Here's how the part is built. I have some questions about the finished solid (model axes, mm). A direction names the side the tool comes from. Coordinates: 2 decimals unless noted, no trailing zeros. Order: outer loops, then holes, each group sorted by start corner. A loop starts at its lowest first (then second) coordinate and runs counter-clockwise, first axis right, second up. Notation, with made-up numbers: (-12, 89) - (43, 89) arc R16 ccw to (43, 115) - close; hole circle Ø11 at (-31, 43.5). An arc over 180 degrees is marked (long way). Answer in a Markdown table with one row per item. Add a question column.
Item 1: I want a section at A-A (z = 113). Please give me the cut outline in (x, y).
Item 2: If I drill on line 1 along Z through (x, y) = (14.5, -1.5); line 2 along X through (y, z) = (-8.75, 84.4); line 3 along Y through (x, z) = (17.5, 31), over which ranges is the centre line in solid material (lowest first)? Write a range as from..to.
Item 3: Will these pins go through, and if not, where does the flat tip stop? pin 1 Ø3 at (x, y) = (15.75, -16.25) entering from +Z; pin 2 Ø5 at (x, y) = (19, 11) entering from +Z; pin 3 Ø6.5 at (x, z) = (13, 97.5) entering from +Y.
Item 4: On a 3-axis mill with a long thin cutter (end or side, diameter ignored), from which of +Z, -Z, +X, -X, +Y, -Y can I reach the whole of each face in a straight line? I mean faces 4 (the cylindrical face through (15.33, 6.297, -72.859)), 5 (the cylindrical face through (20.01, 17.95, 70.2)), 6 (the flat face through (14, 11.5, -65)), 7 (the flat face through (23.028, 20.996, -104.866)). Say none if no direction works.
Item 5: Thinking about a two-plate mould opening in Z: for faces 1 (the flat face through (15.5, 12, 102)), 2 (the cylindrical face through (22.972, 23.75, 76.245)), 3 (the flat face through (16, 2, 130)), which applies, +Z half, -Z half, draft (parallel to the pull), parting line (faces both ways), or undercut?
```python
from build123d import *

# Parameters (mm, degrees)
BOSS_EXTRUDE1_DEPTH      = 25
CUT_EXTRUDE1_DEPTH       = 4
FILLET1_R                = 4
FILLET2_R                = 10
FILLET3_R                = 5
FILLET4_R                = 3
BOSS_EXTRUDE2_DEPTH      = 3
BOSS_EXTRUDE2_DEPTH_BACK = 3
FILLET5_R                = 3
SKETCH6_W                = 13
SKETCH6_H                = 14
BOSS_EXTRUDE3_DEPTH      = 20
BOSS_EXTRUDE4_DEPTH      = 20
SKETCH9_W                = 13
SKETCH9_H                = 2
BOSS_EXTRUDE5_DEPTH      = 8
SKETCH7_W                = 13
SKETCH7_H                = 2
CUT_EXTRUDE2_DEPTH       = 5
SKETCH11_R               = 1.6
CUT_EXTRUDE3_DEPTH       = 19
CUT_EXTRUDE4_START       = -2
SKETCH12_R               = 1.6
CUT_EXTRUDE4_DEPTH       = 2
CUT_EXTRUDE5_DEPTH       = 6.5
CUT_EXTRUDE5_DEPTH_BACK  = 6.5
LARGE_START              = -17
SKETCH15_R               = 6.5
LARGE_SCREW_HOLES_DEPTH  = 17
SKETCH17_W               = 9.5
SKETCH17_H               = 262.988655448
CUT_EXTRUDE6_DEPTH       = 141.64583179
SKETCH18_W               = 3
SKETCH18_H               = 20
CUT_EXTRUDE7_DEPTH       = 203.440732067


with BuildPart() as part:
    # Sketch1 → Boss-Extrude1 (new body)
    with BuildSketch(Plane(origin=(0, 0, 0), x_dir=(0, 0, -1), z_dir=(1, 0, 0))):
        Polygon((0, 0), (-130, 0), (-130, 5), (-100.000366453, 5.148280317), (-77.868517379, 27.5), (101.088229162, 27.5), (114, 18), (114, 0), (74, 0), (74, 7.5), (0, 7.5), align=None)
    extrude(amount=BOSS_EXTRUDE1_DEPTH)

    # Sketch4 → Cut-Extrude1 (cut)
    with BuildSketch(Plane(origin=(25, 0, 0), x_dir=(0, 0, -1), z_dir=(1, 0, 0))):
        Polygon((-100.876178749, 0), (0, 0), (111, 0), (111, 3), (111, 16.482758557), (100.103496394, 24.5), (-76.617181678, 24.5), align=None)
    cut_extrude1 = extrude(amount=-CUT_EXTRUDE1_DEPTH, mode=Mode.SUBTRACT)

    # Mirror2: Cut-Extrude1 across plane
    add(cut_extrude1.mirror(Plane(origin=(12.5, 0, 0), x_dir=(0, 0, 1), z_dir=(1, 0, 0))), mode=Mode.SUBTRACT)

    # Fillet1
    fillet1_edges = [part.edges().sort_by_distance(p)[0] for p in [
        (12.5, 7.5, -74),
        (12.5, 7.5, 0),
    ]]
    fillet(fillet1_edges, radius=FILLET1_R)

    # Fillet2
    fillet2_edges = [part.edges().sort_by_distance(p)[0] for p in [
        (23, 0, 100.876178749),
        (23, 24.5, 76.617181678),
        (23, 24.5, -100.103496394),
        (23, 16.482758557, -111),
        (2, 0, 100.876178749),
        (2, 16.482758557, -111),
        (2, 24.5, -100.103496394),
        (2, 24.5, 76.617181678),
    ]]
    fillet(fillet2_edges, radius=FILLET2_R)

    # Fillet3
    fillet3_edges = [part.edges().sort_by_distance(p)[0] for p in [
        (12.5, 5.148280317, 100.000366453),
        (12.5, 27.5, 77.868517379),
        (12.5, 27.5, -101.088229162),
        (12.5, 18, -114),
    ]]
    fillet(fillet3_edges, radius=FILLET3_R)

    # Fillet4
    fillet4_edges = [part.edges().sort_by_distance(p)[0] for p in [
        (0, 2.5, 130),
        (25, 2.5, 130),
    ]]
    fillet(fillet4_edges, radius=FILLET4_R)

    # Sketch5 → Boss-Extrude2 (add, two sides: drawn at the far end of the back side and taken through both)
    with BuildSketch(Plane(origin=(12.5, 0, 0), x_dir=(0, 0, -1), z_dir=(1, 0, 0)).offset(-BOSS_EXTRUDE2_DEPTH_BACK)):
        Polygon((-117.8659777, 5.059975288), (-103.793914836, 19.271838176), (-72.605250228, 19.271838176), (-95.8659777, 5.059975288), align=None)
    extrude(amount=BOSS_EXTRUDE2_DEPTH + BOSS_EXTRUDE2_DEPTH_BACK)

    # Fillet5
    fillet5_edges = [part.edges().sort_by_distance(p)[0] for p in [
        (12.5, 19.271838176, 103.793914836),
    ]]
    fillet(fillet5_edges, radius=FILLET5_R)

    # Sketch6 → Boss-Extrude3 (add)
    with BuildSketch(Plane.XZ):
        Polygon((0, -111), (4, -111), (4, -93), (21, -93), (21, -111), (25, -111), (25, -114), (0, -114), align=None)
        with Locations((12.5, -102)):
            Rectangle(SKETCH6_W, SKETCH6_H, mode=Mode.SUBTRACT)
    extrude(amount=BOSS_EXTRUDE3_DEPTH)

    # Sketch8 → Boss-Extrude4 (add)
    with BuildSketch(Plane.XZ):
        Polygon((21, 85), (4, 85), (4, 64), (6, 64), (6, 83), (19, 83), (19, 64), (21, 64), align=None)
    extrude(amount=BOSS_EXTRUDE4_DEPTH)

    # Sketch9 → Boss-Extrude5 (add)
    with BuildSketch(Plane.XZ):
        with Locations((12.5, 65)):
            Rectangle(SKETCH9_W, SKETCH9_H)
    extrude(amount=BOSS_EXTRUDE5_DEPTH)

    # Sketch7 → Cut-Extrude2 (cut)
    with BuildSketch(Plane.XZ.offset(20)):
        with Locations((12.5, -94)):
            Rectangle(SKETCH7_W, SKETCH7_H)
    extrude(amount=-CUT_EXTRUDE2_DEPTH, mode=Mode.SUBTRACT)

    # Sketch11 → Cut-Extrude3 (cut)
    with BuildSketch(Plane(origin=(0, 0, -114), x_dir=(-1, 0, 0), z_dir=(0, 0, -1))):
        with Locations((-15.75, -16.25)):
            Circle(SKETCH11_R)
        with Locations((-15.75, -8.75)):
            Circle(SKETCH11_R)
        with Locations((-9.25, -8.75)):
            Circle(SKETCH11_R)
        with Locations((-9.25, -16.25)):
            Circle(SKETCH11_R)
    extrude(amount=-CUT_EXTRUDE3_DEPTH, mode=Mode.SUBTRACT)

    # Sketch12 → Cut-Extrude4 (cut)
    with BuildSketch(Plane.XY.offset(85).offset(CUT_EXTRUDE4_START)):
        with Locations(Location((15.75, -16.25, 0), (0, 0, 180))):
            Circle(SKETCH12_R)
        with Locations(Location((9.25, -16.25, 0), (0, 0, 180))):
            Circle(SKETCH12_R)
        with Locations(Location((9.25, -8.75, 0), (0, 0, 180))):
            Circle(SKETCH12_R)
        with Locations(Location((15.75, -8.75, 0), (0, 0, 180))):
            Circle(SKETCH12_R)
    extrude(amount=CUT_EXTRUDE4_DEPTH, mode=Mode.SUBTRACT)

    # Sketch14 → Cut-Extrude5 (cut, two sides: drawn at the far end of the back side and taken through both)
    with BuildSketch(Plane(origin=(12.5, 0, 0), x_dir=(0, 0, -1), z_dir=(1, 0, 0)).offset(-CUT_EXTRUDE5_DEPTH_BACK)):
        Polygon((-83, 0), (-83, 13.475167258), (-72.975167258, 23.5), (95.592427597, 23.5), (109, 10.092427597), (109, 0), (95, 0), (95, 3.57939317), (87.07939317, 11.5), (-5.825100808, 11.5), (-13.325100808, 4), (-66, 4), (-66, 0), align=None)
    extrude(amount=CUT_EXTRUDE5_DEPTH + CUT_EXTRUDE5_DEPTH_BACK, mode=Mode.SUBTRACT)

    # Sketch15 → large screw holes (cut)
    with BuildSketch(Plane.ZY.offset(-4).offset(LARGE_START)):
        with Locations((-91, 16)):
            Circle(SKETCH15_R)
        with Locations((-39.333333333, 16)):
            Circle(SKETCH15_R)
        with Locations((64, 16)):
            Circle(SKETCH15_R)
        with Locations((12.333333333, 16)):
            Circle(SKETCH15_R)
    extrude(amount=LARGE_SCREW_HOLES_DEPTH, mode=Mode.SUBTRACT)

    # Sketch17 → Cut-Extrude6 (cut, through all)
    with BuildSketch(Plane(origin=(0, 27.5, 0), x_dir=(1, 0, 0), z_dir=(0, 1, 0))):
        with Locations((4.75, -2.000036068)):
            Rectangle(SKETCH17_W, SKETCH17_H)
    extrude(amount=-CUT_EXTRUDE6_DEPTH, mode=Mode.SUBTRACT)

    # Sketch18 → Cut-Extrude7 (cut, through all)
    with BuildSketch(Plane.XY.offset(85)):
        with Locations((11, -10)):
            Rectangle(SKETCH18_W, SKETCH18_H)
    extrude(amount=-CUT_EXTRUDE7_DEPTH, mode=Mode.SUBTRACT)


solid = part.part
```
Values follow:
| question | item | result |
|---|---|---|
| 1 | outline | (9.5, 0) - (25, 0) - (25, 5.08) - (15.5, 5.08) - (15.5, 9.97) - (9.5, 9.97) - close |
| 2 | line 1 | z = -114..-109, -95..-93, 64..66, 83..85 |
| 2 | line 2 | x = 12.5..14.15, 17.35..21 |
| 2 | line 3 | y = 0..4, 23.5..27.5 |
| 3 | pin 1 | stops at z = -93 |
| 3 | pin 2 | stops at z = 96.68 |
| 3 | pin 3 | stops at y = 19.27 |
| 4 | face 4 | +X, -X, -Y |
| 4 | face 5 | +X, -X |
| 4 | face 6 | -X |
| 4 | face 7 | +X, -Y |
| 5 | face 1 | draft |
| 5 | face 2 | undercut |
| 5 | face 3 | +Z half |
